```python
from build123d import *

# Parameters (mm, degrees)
SKETCH1_R           = 40
BOSS_EXTRUDE1_DEPTH = 10
SKETCH2_R           = 52.5
CUT_EXTRUDE1_DEPTH  = 5
SKETCH3_R           = 50
BOSS_EXTRUDE2_DEPTH = 10
BOSS_EXTRUDE3_DEPTH = 20


with BuildPart() as part:
    # Sketch1 → Boss-Extrude1 (new body)
    with BuildSketch(Plane.XY):
        with BuildLine():
            Line((0, 60), (200, 60))
            ThreePointArc((200, 60), (260, 0), (200, -60))
            Line((200, -60), (0, -60))
            ThreePointArc((0, -60), (-60, 0), (0, 60))
        make_face()
        Circle(SKETCH1_R, mode=Mode.SUBTRACT)
    extrude(amount=BOSS_EXTRUDE1_DEPTH)

    # Sketch2 → Cut-Extrude1 (cut)
    with BuildSketch(Plane(origin=(0, 0, 0), x_dir=(-1, 0, 0), z_dir=(0, 0, -1))):
        Circle(SKETCH2_R)
    extrude(amount=-CUT_EXTRUDE1_DEPTH, mode=Mode.SUBTRACT)

    # Sketch3 → Boss-Extrude2 (add)
    with BuildSketch(Plane.XY.offset(10)):
        with BuildLine():
            ThreePointArc((0, -60), (42.426406871, -42.426406871), (60, 0))
            ThreePointArc((60, 0), (42.426406871, 42.426406871), (0, 60))
            ThreePointArc((0, 60), (-60, 0), (0, -60))
        make_face()
        Circle(SKETCH3_R, mode=Mode.SUBTRACT)
    extrude(amount=BOSS_EXTRUDE2_DEPTH)

    # Sketch4 → Boss-Extrude3 (add)
    with BuildSketch(Plane.XY.offset(10)):
        with BuildLine():
            Line((0, -60), (200, -60))
            ThreePointArc((200, -60), (260, 0), (200, 60))
            Line((200, 60), (0, 60))
            ThreePointArc((0, 60), (-60, 0), (0, -60))
        make_face()
        with BuildLine():
            Line((0, -50), (200, -50))
            ThreePointArc((200, -50), (250, 0), (200, 50))
            Line((200, 50), (0, 50))
            ThreePointArc((0, 50), (-50, 0), (0, -50))
        make_face(mode=Mode.SUBTRACT)
    extrude(amount=BOSS_EXTRUDE3_DEPTH)


solid = part.part
```
Build history of the part. All positions in model axes, mm. A direction names the side the tool comes from. Round coordinates to 2 decimals unless told otherwise and drop trailing zeros. Write each loop counter-clockwise with the first axis right and the second up, starting at its lowest first coordinate (ties: lowest second). Pieces come first, ordered by that corner, then holes.
1) Band-saw the part on A-A, the plane z = 25.5. List the corners of the cut face in (x, y).
2) Band-saw the part on C-C, the plane x = -17.5. List the corners of the cut face in (y, z).
3) Pin check, flat tips, straight feed: pin 1 (12 mm diameter, centred on x = 49.5, y = -37, fed in from +Z); pin 2 (8 mm diameter, centred on y = 28, z = 20.5, fed in from -X); pin 3 (3 mm diameter, centred on y = -30.5, z = 11, fed in from -X); pin 4 (12 mm diameter, centred on x = 86.5, y = -30, fed in from -Z). Stop position of each tip, or through.
4) Mould opens along Y. For faces 4 (the cylindrical face through (-49.95, 2.2, 17.64)), 5 (the flat face through (50, 4, 20)), 6 (the flat face through (99, -53, 30)), 7 (the flat face through (101, 60, 15)) say: +Y half, -Y half, draft (parallel to the pull), parting line (faces both ways), or undercut.
5) Band-saw the part on B-B, the plane y = 16.5. List the corners of the cut face in (x, z).
6) Drill centre lines: probe 1 along X at (y, z) = (0, 26.25); probe 2 along X at (y, z) = (-1, 4.75); probe 3 along Y at (x, z) = (0, 7.15). Where is each one in solid material? Low to high.
7) Band-saw the part on D-D, the plane x = 92. List the corners of the cut face in (y, z).
8) 3-axis set-ups, long thin cutter, end or side, ignore diameter. For faces 1 (the flat face through (143, 1, 10)), 2 (the flat face through (12, -39, 5)), 3 (the cylindrical face through (259.985, -1.319, 14.79)): which of +Z, -Z, +X, -X, +Y, -Y reach the whole face in a straight line?
Ans:
1. outline: (0, -60) - (200, -60) arc R60 ccw to (200, 60) - (0, 60) arc R60 ccw to start; hole (0, -50) - (200, -50) arc R50 ccw to (200, 50) - (0, 50) arc R50 ccw to start
2. outline: (-57.39, 0) - (-49.5, 0) - (-49.5, 5) - (-35.97, 5) - (-35.97, 10) - (-46.84, 10) - (-46.84, 30) - (-57.39, 30) - close; (35.97, 5) - (49.5, 5) - (49.5, 0) - (57.39, 0) - (57.39, 30) - (46.84, 30) - (46.84, 10) - (35.97, 10) - close
3. pin 1: stops at z = 20
3. pin 2: stops at x = -54.99
3. pin 3: stops at x = -52.53
3. pin 4: stops at z = 0
4. face 4: undercut
4. face 5: undercut
4. face 6: draft
4. face 7: +Y half
5. outline: (-57.69, 0) - (-49.84, 0) - (-49.84, 5) - (-36.44, 5) - (-36.44, 10) - (-47.2, 10) - (-47.2, 30) - (-57.69, 30) - close; (36.44, 5) - (49.84, 5) - (49.84, 0) - (257.69, 0) - (257.69, 30) - (247.2, 30) - (247.2, 10) - (57.69, 10) - (57.69, 20) - (47.2, 20) - (47.2, 10) - (36.44, 10) - close
6. probe 1: x = -60 to -50, 250 to 260
6. probe 2: x = -59.99 to -52.49, 52.49 to 259.99
6. probe 3: y = -60 to -40, 40 to 60
7. outline: (-60, 0) - (60, 0) - (60, 30) - (50, 30) - (50, 10) - (-50, 10) - (-50, 30) - (-60, 30) - close
8. face 1: +Z
8. face 2: -Z
8. face 3: +Z, -Z, +X
